from build123d import *

# Parameters (mm, degrees)
BOSS_EXTRUDE4_DEPTH = 50
SKETCH5_R           = 1.5
SKETCH5_W           = 7
SKETCH5_H           = 5
SKETCH5_W_2         = 12
CUT_EXTRUDE1_DEPTH  = 65.314778352


with BuildPart() as part:
    # Sketch4 → Boss-Extrude4 (new body)
    with BuildSketch(Plane.XY):
        with BuildLine():
            Line((-1.5, -15.5), (-1.5, 15.5))
            ThreePointArc((-1.5, 15.5), (0.101399131, 19.727512771), (4.260080705, 21.5))
            Line((4.260080705, 21.5), (16.260080705, 21.5))
            Line((16.260080705, 21.5), (16.260080705, 18.5))
            Line((16.260080705, 18.5), (4.260080705, 18.5))
            ThreePointArc((4.260080705, 18.5), (2.265546552, 17.649902138), (1.497503795, 15.622356038))
            Line((1.497503795, 15.622356038), (1.5, 15.5))
            Line((1.5, 15.5), (1.5, -15.5))
            ThreePointArc((1.5, -15.5), (5.823127548, -25.936953157), (16.260080705, -30.260080705))
            Line((16.260080705, -30.260080705), (21.525154636, -30.260080705))
            Line((21.525154636, -30.260080705), (21.525154636, -33.260080705))
            Line((21.525154636, -33.260080705), (16.260080705, -33.260080705))
            ThreePointArc((16.260080705, -33.260080705), (3.701807204, -28.058273501), (-1.5, -15.5))
        make_face()
    extrude(amount=BOSS_EXTRUDE4_DEPTH)

    # Sketch5 → Cut-Extrude1 (cut, through all)
    with BuildSketch(Plane.ZY.offset(1.5)):
        with Locations((28, -0.5)):
            Circle(SKETCH5_R)
        with Locations((22.5, -0.7)):
            Rectangle(SKETCH5_W, SKETCH5_H)
        with Locations((26, 8.3)):
            Rectangle(SKETCH5_W_2, SKETCH5_H)
    extrude(amount=-CUT_EXTRUDE1_DEPTH, mode=Mode.SUBTRACT)


solid = part.part
Design review of the part built by this model. Coordinates are the model's own, in mm. A direction names the side the tool comes from. Give positions to 0.01 mm unless a question says otherwise; leave off trailing zeros. Order: outer loops, then holes, each group sorted by start corner. A loop starts at its lowest first (then second) coordinate and runs counter-clockwise, first axis right, second up. Notation, with made-up numbers: (3, 16) - (22, 16) arc R19 ccw to (22, 39) - close; hole circle Ø1 at (32, 18.25). An arc over 180 degrees is marked (long way). Use CSV: the item, a comma, the result in double quotes. Start each with the question number.
Q1. Take a section at D-D (x = 14.25). State the section outline as (y, z) points.
Q2. For P1, Ø3.5, axis at x = 11.5, z = 32, coming from the -Y side; P2, Ø1.5, axis at x = 0.5, z = 21, coming from the +Y side; P3, Ø2.5, axis at x = 18.5, z = 31.5, coming from the +Y side; P4, Ø12, axis at x = 4, y = -16.5, coming from the -Z side, all flat-tipped, find the tip position at first contact; note any pin that passes through.
Q3. Take a section at B-B (z = 28). State the section outline as (x, y) points, and give its area (3 significant figures).
Q4. Take a section at C-C (y = 10). State the section outline as (x, z) points, and give its area (3 significant figures).
Q5. Machinability: for faces 1 (the face through (-1.5, -4, 25)), 2 (the face through (16.26, 20, 25)), 3 (the face through (10, 18.5, 25)), 4 (the face through (0, 10.8, 26)), which of the approach directions +Z, -Z, +X, -X, +Y, -Y give a long, thin tool a straight path to every point of the face, cutting with its end or side? Answer none if there is none.
Q6. Take a section at A-A (y = -0.5). State the section outline as (x, z) points.
Q7. For line 1 (X direction, y = -14, z = 13); line 2 (Y direction, x = 0, z = 28); line 3 (Y direction, x = 18, z = 23), list the stretches that pass through material, from the lowest coordinate up.
Q8. Draft analysis for pull direction Z (two halves, no side actions). For faces 5 (the face through (1, -4, 50)), 6 (the face through (10, 21.5, 25)), 7 (the face through (1, -4, 0)), 8 (the face through (-0.02, -0.43, 26.5)), state which applies: pulls with the +Z half, pulls with the -Z half, needs draft (parallel to the pull), parting line crosses it, or undercut.
Calculated:
1,outline,"(-33.15, 0) - (-30.12, 0) - (-30.12, 50) - (-33.15, 50) - close; (18.5, 0) - (21.5, 0) - (21.5, 50) - (18.5, 50) - close"
2,P1,"stops at y = -33"
2,P2,"stops at y = 20.65"
2,P3,"stops at y = -30.26"
2,P4,"stops at z = 0"
3,outline,"(-1.5, -15.5) arc R17.76 ccw to (16.26, -33.26) - (21.53, -33.26) - (21.53, -30.26) - (16.26, -30.26) arc R14.76 cw to (1.5, -15.5) - (1.5, -2) - (-1.5, -2) - close; (-1.5, 1) - (1.5, 1) - (1.5, 5.8) - (-1.5, 5.8) - close; (-1.5, 10.8) - (1.5, 10.8) - (1.5, 15.5) - (1.5, 15.62) arc R2.76 cw to (4.26, 18.5) - (16.26, 18.5) - (16.26, 21.5) - (4.26, 21.5) arc R5.76 ccw to (-1.5, 15.5) - close"
3,area,"218 mm²"
4,outline,"(-1.5, 0) - (1.5, 0) - (1.5, 20) - (-1.5, 20) - close; (-1.5, 32) - (1.5, 32) - (1.5, 50) - (-1.5, 50) - close"
4,area,"114 mm²"
5,face 1,"+Z, -Z, -X, +Y, -Y"
5,face 2,"+Z, -Z, +X, +Y"
5,face 3,"+Z, -Z, +X"
5,face 4,"+X, -X"
6,outline,"(-1.5, 0) - (1.5, 0) - (1.5, 19) - (-1.5, 19) - close; (-1.5, 26) - (1.5, 26) - (1.5, 26.5) - (-1.5, 26.5) - close; (-1.5, 29.5) - (1.5, 29.5) - (1.5, 50) - (-1.5, 50) - close"
7,line 1,"x = -1.5 to 1.5"
7,line 2,"y = -22.64 to -2, 1 to 5.8, 10.8 to 19.62"
7,line 3,"y = -33.26 to -30.26"
8,face 5,"pulls with the +Z half"
8,face 6,"needs draft"
8,face 7,"pulls with the -Z half"
8,face 8,"undercut"
